```python
from build123d import *

# Parameters (mm, degrees)
SKETCH1_R           = 11
BOSS_EXTRUDE1_DEPTH = 7
SKETCH2_W           = 5
SKETCH2_H           = 2.5
BOSS_EXTRUDE2_DEPTH = 13
CHAMFER2_SIZE       = 2
BOSS_EXTRUDE6_DEPTH = 2.5
CHAMFER3_SIZE       = 2
CHAMFER4_SIZE       = 2
BOSS_EXTRUDE4_DEPTH = 2.5
CHAMFER6_SIZE       = 2.5
CHAMFER7_SIZE       = 7
CHAMFER7_SIZE_2     = 13.165085257


with BuildPart() as part:
    # Sketch1 → Boss-Extrude1 (new body)
    with BuildSketch(Plane.XY):
        Polygon((-15, 11.5), (-12.5, 14), (12.5, 14), (15, 11.5), (15, -14), (-15, -14), align=None)
        Circle(SKETCH1_R, mode=Mode.SUBTRACT)
    extrude(amount=BOSS_EXTRUDE1_DEPTH)

    # Sketch2 → Boss-Extrude2 (add)
    with BuildSketch(Plane(origin=(0, 0, 0), x_dir=(-1, 0, 0), z_dir=(0, 0, -1))):
        with Locations((-12.5, -12.75)):
            Rectangle(SKETCH2_W, SKETCH2_H)
        with Locations((12.5, -12.75)):
            Rectangle(SKETCH2_W, SKETCH2_H)
    extrude(amount=BOSS_EXTRUDE2_DEPTH)

    # Chamfer2
    chamfer2_edges = [part.edges().sort_by_distance(p)[0] for p in [
        (-10, -12.75, 0),
        (10, -12.75, 0),
    ]]
    chamfer(chamfer2_edges, length=CHAMFER2_SIZE)

    # Sketch5 → Boss-Extrude6 (add)
    with BuildSketch(Plane.XZ.offset(14)):
        Polygon((-10, -2), (-10, -7.5), (10, -7.5), (10, -2), (8, 0), (-8, 0), align=None)
    extrude(amount=-BOSS_EXTRUDE6_DEPTH)

    # Chamfer3
    chamfer3_edges = [part.edges().sort_by_distance(p)[0] for p in [
        (15, -1.25, 7),
    ]]
    chamfer(chamfer3_edges, length=CHAMFER3_SIZE)

    # Chamfer4
    chamfer4_edges = [part.edges().sort_by_distance(p)[0] for p in [
        (-15, -1.25, 7),
    ]]
    chamfer(chamfer4_edges, length=CHAMFER4_SIZE)

    # Sketch4 → Boss-Extrude4 (add)
    with BuildSketch(Plane(origin=(0, 0, 0), x_dir=(-1, 0, 0), z_dir=(0, 0, -1))):
        Polygon((-15, -1.25), (15, 11.5), (12.5, 14), (-12.5, 14), (-15, 11.5), align=None)
    extrude(amount=BOSS_EXTRUDE4_DEPTH)

    # Chamfer6
    # the kernel refuses this chamfer: 2.5 mm, written as the material it adds along each edge
    with BuildSketch(Plane(origin=(20.916998416, -3.764724327, 0), x_dir=(-0.39099275668343275, -0.9199829569021947, 0.02749587661058635), z_dir=(-0.9203309184584746, 0.39114064034485174, 0))) as chamfer6_piece_1_section:
        Polygon((CHAMFER6_SIZE * 0.999621916911, -CHAMFER6_SIZE * 0.0274958766106), (-CHAMFER6_SIZE * 0.0274958766106, -CHAMFER6_SIZE * 0.999621916911), (0, 0), align=None)
    chamfer6_piece_1 = extrude(amount=17.214861222, mode=Mode.PRIVATE)
    chamfer6_piece_1 = chamfer6_piece_1 - Plane(origin=(0, 0, -0.830769879), x_dir=(1, 0, 0), z_dir=(0, 0, -1)) * Cylinder(11, 45, mode=Mode.PRIVATE)
    chamfer6_piece_1 = split(chamfer6_piece_1, bisect_by=Plane(origin=(15, -1.305255327, -0.830769879), z_dir=(-1, 0, 0)), keep=Keep.TOP, mode=Mode.PRIVATE)
    add(chamfer6_piece_1)
    with BuildSketch(Plane(origin=(-1.383846422, 5.71313473, 0), x_dir=(-0.39099275668343275, -0.9199829569021946, 0.02749587661058637), z_dir=(-0.9203309184584746, 0.39114064034485174, 0))) as chamfer6_piece_2_section:
        Polygon((CHAMFER6_SIZE * 0.999621916911, -CHAMFER6_SIZE * 0.0274958766106), (-CHAMFER6_SIZE * 0.0274958766106, -CHAMFER6_SIZE * 0.999621916911), (0, 0), align=None)
    chamfer6_piece_2 = extrude(amount=21.224052785, mode=Mode.PRIVATE)
    chamfer6_piece_2 = chamfer6_piece_2 - Plane(origin=(0, 0, -0.851096237), x_dir=(1, 0, 0), z_dir=(0, 0, -1)) * Cylinder(11, 53, mode=Mode.PRIVATE)
    chamfer6_piece_2 = split(chamfer6_piece_2, bisect_by=Plane(origin=(-15, 9.126408424, -0.851096237), z_dir=(1, 0, 0)), keep=Keep.TOP, mode=Mode.PRIVATE)
    add(chamfer6_piece_2)

    # Chamfer7
    # the kernel refuses this chamfer: 13.165085257, 7 mm, written as the material it adds along each edge
    with BuildSketch(Plane(origin=(-15, -11.5, 0), x_dir=(0, 0.9979482451756082, 0.06402577567608186), z_dir=(1, 0, 0))) as chamfer7_piece_1_section:
        Polygon((CHAMFER7_SIZE * 0.997948245176, -CHAMFER7_SIZE * 0.0640257756761), (-CHAMFER7_SIZE_2 * 0.0640257756781, -CHAMFER7_SIZE_2 * 0.997948245208), (0, 0), align=None)
    chamfer7_piece_1 = extrude(amount=30, mode=Mode.PRIVATE)
    chamfer7_piece_1 = chamfer7_piece_1 - Plane(origin=(0, 0, -3.073682767), x_dir=(1, 0, 0), z_dir=(0, 0, -1)) * Cylinder(11, 113, mode=Mode.PRIVATE)
    chamfer7_piece_1 = split(chamfer7_piece_1, bisect_by=Plane(origin=(-12.500128058, -8.887755394, -7.5), z_dir=(0, 0, 1)), keep=Keep.TOP, mode=Mode.PRIVATE)
    chamfer7_piece_1 = split(chamfer7_piece_1, bisect_by=Plane(origin=(-10, -8.887755394, -3.073682767), z_dir=(-1, 0, 0)), keep=Keep.TOP, mode=Mode.PRIVATE)
    add(chamfer7_piece_1)
    with BuildSketch(Plane(origin=(-15, -11.5, 0), x_dir=(0, 0.9979482451756082, 0.06402577567608186), z_dir=(1, 0, 0))) as chamfer7_piece_2_section:
        Polygon((CHAMFER7_SIZE * 0.997948245176, -CHAMFER7_SIZE * 0.0640257756761), (-CHAMFER7_SIZE_2 * 0.0640257756781, -CHAMFER7_SIZE_2 * 0.997948245208), (0, 0), align=None)
    chamfer7_piece_2 = extrude(amount=30, mode=Mode.PRIVATE)
    chamfer7_piece_2 = split(chamfer7_piece_2, bisect_by=Plane(origin=(-12.5, -10.721530873, -7.5), z_dir=(0, 0, -1)), keep=Keep.TOP, mode=Mode.PRIVATE)
    chamfer7_piece_2 = split(chamfer7_piece_2, bisect_by=Plane(origin=(-10, -10.721530873, -9.597564575), z_dir=(-1, 0, 0)), keep=Keep.TOP, mode=Mode.PRIVATE)
    chamfer7_piece_2 = split(chamfer7_piece_2, bisect_by=Plane(origin=(-12.5, -10.721530873, -13), z_dir=(0, 0, 1)), keep=Keep.TOP, mode=Mode.PRIVATE)
    add(chamfer7_piece_2)
    with BuildSketch(Plane(origin=(-15, -11.5, 0), x_dir=(0, 0.9979482451756082, 0.06402577567608186), z_dir=(1, 0, 0))) as chamfer7_piece_3_section:
        Polygon((CHAMFER7_SIZE * 0.997948245176, -CHAMFER7_SIZE * 0.0640257756761), (-CHAMFER7_SIZE_2 * 0.0640257756781, -CHAMFER7_SIZE_2 * 0.997948245208), (0, 0), align=None)
    chamfer7_piece_3 = extrude(amount=30, mode=Mode.PRIVATE)
    chamfer7_piece_3 = chamfer7_piece_3 - Plane(origin=(0, 0, -3.793876077), x_dir=(1, 0, 0), z_dir=(0, 0, -1)) * Cylinder(11, 113, mode=Mode.PRIVATE)
    chamfer7_piece_3 = split(chamfer7_piece_3, bisect_by=Plane(origin=(-9.499486782, -6.598719884, -7.5), z_dir=(0, 0, 1)), keep=Keep.TOP, mode=Mode.PRIVATE)
    chamfer7_piece_3 = split(chamfer7_piece_3, bisect_by=Plane(origin=(10, -6.598719884, -3.793876077), z_dir=(-1, 0, 0)), keep=Keep.TOP, mode=Mode.PRIVATE)
    chamfer7_piece_3 = split(chamfer7_piece_3, bisect_by=Plane(origin=(-10, -6.598719884, -3.793876077), z_dir=(1, 0, 0)), keep=Keep.TOP, mode=Mode.PRIVATE)
    add(chamfer7_piece_3)
    with BuildSketch(Plane(origin=(-15, -11.5, 0), x_dir=(0, 0.9979482451756082, 0.06402577567608186), z_dir=(1, 0, 0))) as chamfer7_piece_4_section:
        Polygon((CHAMFER7_SIZE * 0.997948245176, -CHAMFER7_SIZE * 0.0640257756761), (-CHAMFER7_SIZE_2 * 0.0640257756781, -CHAMFER7_SIZE_2 * 0.997948245208), (0, 0), align=None)
    chamfer7_piece_4 = extrude(amount=30, mode=Mode.PRIVATE)
    chamfer7_piece_4 = split(chamfer7_piece_4, bisect_by=Plane(origin=(12.5, -10.721530873, -7.5), z_dir=(0, 0, -1)), keep=Keep.TOP, mode=Mode.PRIVATE)
    chamfer7_piece_4 = split(chamfer7_piece_4, bisect_by=Plane(origin=(10, -10.721530873, -9.597564575), z_dir=(1, 0, 0)), keep=Keep.TOP, mode=Mode.PRIVATE)
    chamfer7_piece_4 = split(chamfer7_piece_4, bisect_by=Plane(origin=(12.5, -10.721530873, -13), z_dir=(0, 0, 1)), keep=Keep.TOP, mode=Mode.PRIVATE)
    add(chamfer7_piece_4)
    with BuildSketch(Plane(origin=(-15, -11.5, 0), x_dir=(0, 0.9979482451756082, 0.06402577567608186), z_dir=(1, 0, 0))) as chamfer7_piece_5_section:
        Polygon((CHAMFER7_SIZE * 0.997948245176, -CHAMFER7_SIZE * 0.0640257756761), (-CHAMFER7_SIZE_2 * 0.0640257756781, -CHAMFER7_SIZE_2 * 0.997948245208), (0, 0), align=None)
    chamfer7_piece_5 = extrude(amount=30, mode=Mode.PRIVATE)
    chamfer7_piece_5 = chamfer7_piece_5 - Plane(origin=(0, 0, -3.073682766), x_dir=(1, 0, 0), z_dir=(0, 0, -1)) * Cylinder(11, 113, mode=Mode.PRIVATE)
    chamfer7_piece_5 = split(chamfer7_piece_5, bisect_by=Plane(origin=(12.500128057, -8.887755394, -7.5), z_dir=(0, 0, 1)), keep=Keep.TOP, mode=Mode.PRIVATE)
    chamfer7_piece_5 = split(chamfer7_piece_5, bisect_by=Plane(origin=(10, -8.887755394, -3.073682766), z_dir=(1, 0, 0)), keep=Keep.TOP, mode=Mode.PRIVATE)
    add(chamfer7_piece_5)


solid = part.part
```
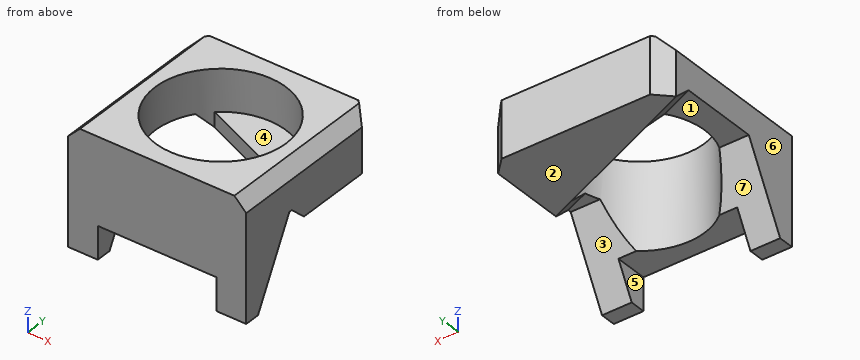
Geometry: final body of the model. Coordinates: model frame, mm. Face numbers are marked on the shaded views. A direction names the side the tool comes from. Give positions to 0.01 mm unless a question says otherwise; leave off trailing zeros. Loops run counter-clockwise (first coordinate to the right, second up) from the corner with the lowest first, then second, coordinate; pieces in that order, holes last. Notation, with made-up numbers: (-19.75, -25) - (4.25, -25) arc R14 cw to (4.25, -7) - close; hole circle Ø9 at (22, 67). An arc over 180 degrees is marked (long way). Answer as CSV lines item,"result". Start each with the question number.
(1) Mould query, pull axis X, two halves, no side actions, for the marked faces 5, 6 and 7. Classes: +X half, -X half, draft (parallel to the pull), parting line (faces both ways), or undercut.
(2) Ray query, line 1 along Y through (x, z) = (0, 5.5); line 2 along X through (y, z) = (0, 2.25); line 3 along X through (y, z) = (2.5, 1.5). Return the intervals inside material, ascending. Write a range as [from, to].
(3) Pin query (flat end, axial travel): P1, Ø3, axis at y = -10, z = -10.5, coming from the -X side; P2, Ø6, axis at y = -3, z = -7.5, coming from the +X side; P3, Ø1.5, axis at x = 2.5, z = -5.5, coming from the +Y side; P4, Ø12, axis at x = 2, y = 9.5, coming from the -Z side. Return the tip coordinate at first contact, or that it passes through.
(4) Section query C-C (x = -6). Output: boundary loops of the cut face in (y, z) (3 decimals), and give its area (3 significant figures).
(5) Section query B-B (y = -6.5). Output: boundary loops of the cut face in (x, z), and give its area (3 significant figures).
(6) Section query A-A (z = 5.75). Output: boundary loops of the cut face in (x, y).
(7) Reachability of the marked faces 1, 2, 3 and 4 from +Z, -Z, +X, -X, +Y, -Y: full face, straight path, thin tool, end or side. Return the list, or none.
(8) Section query D-D (z = -9.5). Output: boundary loops of the cut face in (x, y).
Worked answers:
1,face 5,"undercut"
1,face 6,"-X half"
1,face 7,"draft"
2,line 1,"y = [-14, -11], [11, 14]"
2,line 2,"x = [-15, -11], [11, 15]"
2,line 3,"x = [-15, -10.71], [10.71, 15]"
3,P1,"stops at x = -15"
3,P2,"passes through"
3,P3,"stops at y = -10.51"
3,P4,"stops at z = -2.5"
4,outline,"(-14, -7.5) - (-9.22, -7.5) - (-9.22, 7) - (-14, 7) - close; (7.675, -2.5) - (14, -2.5) - (14, 7) - (9.22, 7) - (9.22, 0) - (7.675, 0) - close"
4,area,"119 mm^2"
5,outline,"(-15, -3.76) - (-8.87, -3.76) - (-8.87, 7) - (-13, 7) - (-15, 5) - close; (8.87, -3.76) - (15, -3.76) - (15, 5) - (13, 7) - (8.87, 7) - close"
5,area,"128 mm^2"
6,outline,"(-14.25, -14) - (14.25, -14) - (14.25, 12.25) - (12.5, 14) - (-12.5, 14) - (-14.25, 12.25) - close; hole circle Ø22 at (0, 0)"
7,face 1,"-Z, -X"
7,face 2,"-Z, +X, -X, +Y"
7,face 3,"-Z, +X, -X"
7,face 4,"+Z"
8,outline,"(-15, -14) - (-10, -14) - (-10, -9.55) - (-15, -9.55) - close; (10, -14) - (15, -14) - (15, -9.55) - (10, -9.55) - close"
